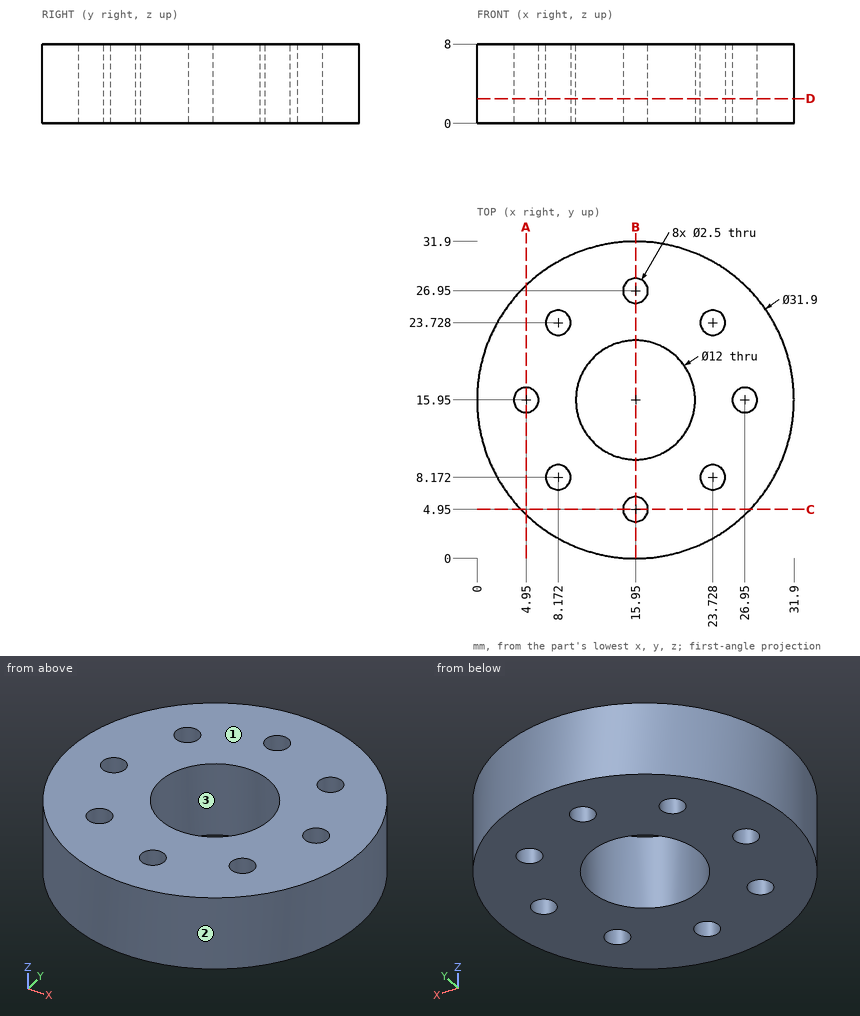
Geometry check sheet. Reference: drawing and pictorial views, mm from the part's lowest x, y, z. Give positions to 0.01 mm unless a question says otherwise; leave off trailing zeros. Loops run counter-clockwise (first coordinate to the right, second up) from the corner with the lowest first, then second, coordinate; pieces in that order, holes last. Notation, with made-up numbers: (29.25, -6) -> (50.25, -6) arc R12 cw to (50.25, 3) -> close; hole circle Ø6 at (84.25, 56). An arc over 180 degrees is marked (long way). Answer in a Markdown table with one row per item. Add a question column.
1) Cross-section at D-D on z = 2.5. State how many separate pieces and enclosed holes the cut face has, and give its area (3 significant figures).
2) Cross-section at A-A on x = 4.95. Record the boundary of the cut face in (y, z), and give its area (3 significant figures).
3) Cross-section at B-B on x = 15.95. Record the boundary of the cut face in (y, z), and give its area (3 significant figures).
4) Material ranges on probe 1 along Y at (x, z) = (15.95, 5.75); probe 2 along Y at (x, z) = (8.5, 5.75) (1 decimal); probe 3 along X at (y, z) = (15, 7) (1 decimal), recorded low to high. Write a range as from..to.
5) Draft check along Y on the marked faces 1, 2 and 3. Enter one of: pulls with the +Y half, pulls with the -Y half, needs draft (parallel to the pull), parting line crosses it, or undercut.
6) Gauge pin test, flat ends, axial feed: P1, Ø2, axis at y = 6.5, z = 4.5, coming from the +X side; P2, Ø4, axis at x = 12.5, z = 5.5, coming from the -Y side; P3, Ø2, axis at x = 23.73, y = 23.73, coming from the +Z side; P4, Ø3, axis at x = 22, z = 5.5, coming from the +Y side. Record the tip position at first contact, or that the pin passes through.
Outcome:
| question | item | result |
|---|---|---|
| 1 | separate pieces | 1 |
| 1 | enclosed holes | 9 |
| 1 | area | 647 mm^2 |
| 2 | outline | (4.4, 0) -> (14.7, 0) -> (14.7, 8) -> (4.4, 8) -> close; (17.2, 0) -> (27.5, 0) -> (27.5, 8) -> (17.2, 8) -> close |
| 2 | area | 165 mm^2 |
| 3 | outline | (0, 0) -> (3.7, 0) -> (3.7, 8) -> (0, 8) -> close; (6.2, 0) -> (9.95, 0) -> (9.95, 8) -> (6.2, 8) -> close; (21.95, 0) -> (25.7, 0) -> (25.7, 8) -> (21.95, 8) -> close; (28.2, 0) -> (31.9, 0) -> (31.9, 8) -> (28.2, 8) -> close |
| 3 | area | 119 mm^2 |
| 4 | probe 1 | y = 0..3.7, 6.2..9.95, 21.95..25.7, 28.2..31.9 |
| 4 | probe 2 | y = 1.8..7, 9.4..22.5, 24.9..30.1 |
| 4 | probe 3 | x = 0..4.1, 5.8..10, 21.9..26.1, 27.8..31.9 |
| 5 | face 1 | needs draft |
| 5 | face 2 | parting line crosses it |
| 5 | face 3 | undercut |
| 6 | P1 | stops at x = 29.48 |
| 6 | P2 | stops at y = 0.07 |
| 6 | P3 | passes through |
| 6 | P4 | stops at y = 31.24 |
